Here's how the part is built. I have some questions about the finished solid (model axes, mm). Round coordinates to 2 decimals unless told otherwise and drop trailing zeros. Order: outer loops, then holes, each group sorted by start corner. A loop starts at its lowest first (then second) coordinate and runs counter-clockwise, first axis right, second up.
```python
from build123d import *

# Parameters (mm, degrees)
SKETCH1_W                = 40
SKETCH1_H                = 40
SKETCH1_W_2              = 34
SKETCH1_H_2              = 34
EXTRUDE_THIN1_DEPTH      = 1200
FILLET1_R                = 0.5
FILLET2_R                = 3
F_8_0_8_DIAMETER_HOLE1_D = 8
SKETCH5_R                = 4
CUT_EXTRUDE1_DEPTH       = 1201.833044182


with BuildPart() as part:
    # Sketch1 → Extrude-Thin1 (new body)
    with BuildSketch(Plane.XY):
        Rectangle(SKETCH1_W, SKETCH1_H)
        Rectangle(SKETCH1_W_2, SKETCH1_H_2, mode=Mode.SUBTRACT)
    extrude(amount=EXTRUDE_THIN1_DEPTH)

    # Fillet1
    fillet1_edges = [part.edges().sort_by_distance(p)[0] for p in [
        (17, -17, 600),
        (17, 17, 600),
        (-17, 17, 600),
        (-17, -17, 600),
    ]]
    fillet(fillet1_edges, radius=FILLET1_R)

    # Fillet2
    fillet2_edges = [part.edges().sort_by_distance(p)[0] for p in [
        (20, -20, 600),
        (-20, -20, 600),
        (-20, 20, 600),
        (20, 20, 600),
    ]]
    fillet(fillet2_edges, radius=FILLET2_R)

    # Ø8.0 (8) Diameter Hole1 (through all)
    with Locations(Plane(origin=(0, 20, 0), x_dir=(1, 0, 0), z_dir=(0, 1, 0))):
        with Locations((0, -20), (0, -1180)):
            Hole(F_8_0_8_DIAMETER_HOLE1_D / 2)

    # Sketch5 → Cut-Extrude1 (cut, through all)
    with BuildSketch(Plane(origin=(0, 20, 0), x_dir=(1, 0, 0), z_dir=(0, 1, 0))):
        with Locations(Location((8, -1075, 0), (0, 0, 270))):
            Circle(SKETCH5_R)
    extrude(amount=-CUT_EXTRUDE1_DEPTH, mode=Mode.SUBTRACT)


solid = part.part
```
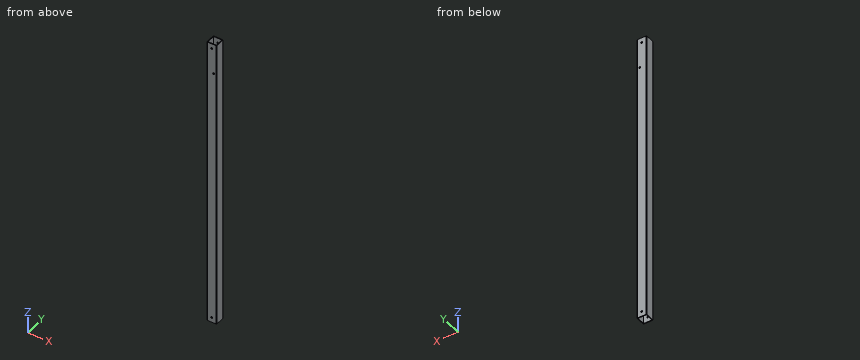
1. If we section it at B-B, the plane y = -7: Write out the boundary of the cut face in (x, z), and give its area (3 significant figures).
Evaluation:
outline: (-20, 0) - (-17, 0) - (-17, 1200) - (-20, 1200) - close; (17, 0) - (20, 0) - (20, 1200) - (17, 1200) - close
area: 7,200 mm2
2. If we section it at A-A, the plane z = 369: Write out the boundary of the cut face in (x, y).
Evaluation:
outline: (-20, -17) arc R3 ccw to (-17, -20) - (17, -20) arc R3 ccw to (20, -17) - (20, 17) arc R3 ccw to (17, 20) - (-17, 20) arc R3 ccw to (-20, 17) - close; hole (-17, -16.5) arc R0.5 ccw to (-16.5, -17) - (16.5, -17) arc R0.5 ccw to (17, -16.5) - (17, 16.5) arc R0.5 ccw to (16.5, 17) - (-16.5, 17) arc R0.5 ccw to (-17, 16.5) - close
3. I'm going to push a flat-ended pin straight in: P1, Ø5, axis at x = 0, z = 20, coming from the -Y side. Where does the tip first touch, or does it pass through?
Evaluation:
P1: passes through
4. I need wall thicknesses on probe 1 along Z at (x, y) = (0, -17.65); probe 2 along Y at (x, z) = (10.5, 607.5); probe 3 along X at (y, z) = (18, 20). Which ranges of each line are inside material? Lowest first, please.
Evaluation:
probe 1: z = 0 to 16, 24 to 1176, 1184 to 1200
probe 2: y = -20 to -17, 17 to 20
probe 3: x = -19.83 to -4, 4 to 19.83
